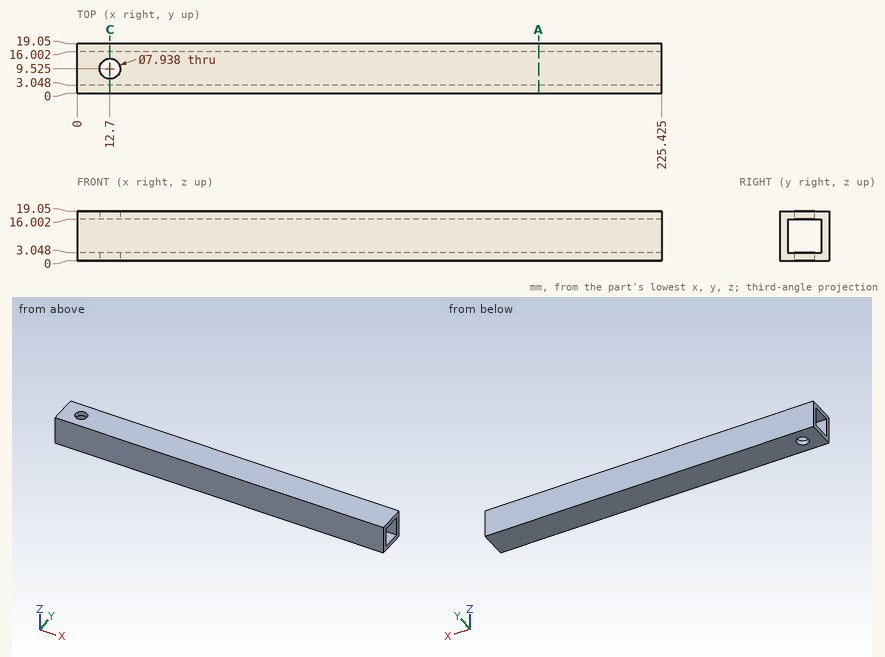
Could you check a few things on this drawing? It's one solid part, dimensions in mm from its lowest x, y, z. Coordinates: 2 decimals unless noted, no trailing zeros. Write each loop counter-clockwise with the first axis right and the second up, starting at its lowest first coordinate (ties: lowest second). Pieces come first, ordered by that corner, then holes. Notation, with made-up numbers: (54, 77) - (86, 77) arc R13 cw to (86, 90) - close; hole circle Ø11 at (22, -29). An arc over 180 degrees is marked (long way). Return JSON: item names as keys, results as strings. Group by question number.
Item 1: Please list where this line runs through material, in increasing order: probe 1 along Y at (x, z) = (93.5, 8).
Item 2: If we section it at C-C (x = 12.7): Write out the boundary of the cut face in (y, z), then the cut area to 3 significant figures.
Item 3: I'm going to push a flat-ended pin straight in: pin 1 Ø4 at (y, z) = (6.5, 7) entering from +X. Where does the tip first touch, or does it pass through?
Item 4: If we section it at A-A (x = 178): Write out the boundary of the cut face in (y, z).
Return value:
{
 "1": {"probe 1": "y = 0 to 3.05, 16 to 19.05"},
 "2": {"outline": "(0, 0) - (5.56, 0) - (5.56, 3.05) - (3.05, 3.05) - (3.05, 16) - (5.56, 16) - (5.56, 19.05) - (0, 19.05) - close; (13.49, 0) - (19.05, 0) - (19.05, 19.05) - (13.49, 19.05) - (13.49, 16) - (16, 16) - (16, 3.05) - (13.49, 3.05) - close", "area": "147 mm^2"},
 "3": {"pin 1": "passes through"},
 "4": {"outline": "(0, 0) - (19.05, 0) - (19.05, 19.05) - (0, 19.05) - close; hole (3.05, 3.05) - (16, 3.05) - (16, 16) - (3.05, 16) - close"}
}
